from build123d import *

# Parameters (mm, degrees)
BORE_DEPTH           = 23.338105056
BORE_DEPTH_BACK      = 23.338105056
SKETCH2_R            = 6.35
RETAINING_HOLE_2_R   = 1.6891
RETAINING_HOLE_DEPTH = 23.338105056
ID_FILLET_R          = 0.254
OD_CHAMFER_SIZE      = 0.254
O_RINGS_2_W          = 1.49225
O_RINGS_2_H          = 1.666875


with BuildPart() as part:
    # Sketch1 → Bearing (revolve)
    with BuildSketch(Plane(origin=(0, 0, 0), x_dir=(0, 0, -1), z_dir=(1, 0, 0)), mode=Mode.PRIVATE) as bearing_sk:
        Polygon((-15.875, 0), (15.875, 0), (15.875, -11.1125), (12.3063, -11.1125), (12.3063, -10.00125), (11.1125, -10.00125), (11.1125, -11.1125), (-11.1125, -11.1125), (-11.1125, -10.00125), (-12.3063, -10.00125), (-12.3063, -11.1125), (-15.875, -11.1125), align=None)
    revolve(bearing_sk.sketch.rotate(Axis((0, 0, 15.875), (0, 0, -1)), 270), axis=Axis((0, 0, 15.875), (0, 0, -1)))

    # Sketch2 → Bore (cut, two sides: drawn at the far end of the back side and taken through both)
    with BuildSketch(Plane.XY.offset(-BORE_DEPTH_BACK)):
        Circle(SKETCH2_R)
    extrude(amount=BORE_DEPTH + BORE_DEPTH_BACK, mode=Mode.SUBTRACT)

    # Retaining Hole 2 → Retaining Hole (cut, through all)
    with BuildSketch(Plane(origin=(0, 0, 0), x_dir=(0, 0, -1), z_dir=(1, 0, 0))):
        with Locations(Location((0, 0, 0), (0, 0, 180))):
            Circle(RETAINING_HOLE_2_R)
    extrude(amount=RETAINING_HOLE_DEPTH, mode=Mode.SUBTRACT)

    # ID Fillet
    id_fillet_edges = [part.edges().sort_by_distance(p)[0] for p in [
        (-6.35, 0, -15.875),
        (-6.35, 0, 15.875),
    ]]
    fillet(id_fillet_edges, radius=ID_FILLET_R)

    # OD Chamfer
    od_chamfer_edges = [part.edges().sort_by_distance(p)[0] for p in [
        (-11.1125, 0, 15.875),
        (-11.1125, 0, -15.875),
    ]]
    chamfer(od_chamfer_edges, length=OD_CHAMFER_SIZE)

    # O-Rings 2 → O-Rings (revolve, cut)
    with BuildSketch(Plane(origin=(0, 0, 0), x_dir=(0, 0, -1), z_dir=(1, 0, 0)), mode=Mode.PRIVATE) as o_rings_sk:
        with Locations((-6.969125, -10.2790625)):
            Rectangle(O_RINGS_2_W, O_RINGS_2_H)
        with Locations((6.969125, -10.2790625)):
            Rectangle(O_RINGS_2_W, O_RINGS_2_H)
    revolve(o_rings_sk.sketch.rotate(Axis((0, 0, 15.875), (0, 0, -1)), 270), axis=Axis((0, 0, 15.875), (0, 0, -1)), mode=Mode.SUBTRACT)


solid = part.part
The model under review builds one solid part; all positions refer to its coordinate system, in mm. A direction names the side the tool comes from. Round coordinates to 2 decimals unless told otherwise and drop trailing zeros. Answer as a JSON object with one key per item and string values.
1. To check wall thickness, follow line 1 along Z through (x, y) = (4.25, 8.75) (3 decimals); line 2 along Z through (x, y) = (2.75, 10) (1 decimal); line 3 along Y through (x, z) = (0.25, -7). State the ranges of each line that lie inside material, in increasing order.
Results found:
{"line 1": "z = -15.875 to -7.715, -6.223 to 6.223, 7.715 to 15.875", "line 2": "z = -15.9 to -12.3, -11.1 to -7.7, -6.2 to 6.2, 7.7 to 11.1, 12.3 to 15.9", "line 3": "y = -9.44 to -6.35, 6.35 to 9.44"}
2. Machinability: for faces 4 (the face through (5.974, -9.37, 9.438)), 5 (the face through (-5, 8.2, 6.223)), 6 (the face through (8.58, 1.5, 0.78)), which of the approach directions +Z, -Z, +X, -X, +Y, -Y give a long, thin tool a straight path to every point of the face, cutting with its end or side? Answer none if there is none.
Results found:
{"face 4": "+Z, -Z", "face 5": "none", "face 6": "+X"}
3. Clearance check with flat-ended pins moving along their axes: pin 1 (8 mm diameter, centred on y = -3.5, z = -7.5, fed in from +X); pin 2 (6 mm diameter, centred on x = -3.5, z = 6, fed in from +Y); pin 3 (1.5 mm diameter, centred on x = 4, z = 8.5, fed in from +Y); pin 4 (1.5 mm diameter, centred on x = -8.5, z = 11, fed in from +Y). State where each tip first meets the part, or that it passes through.
Results found:
{"pin 1": "stops at x = 11.11", "pin 2": "stops at y = 11.1", "pin 3": "stops at y = 10.63", "pin 4": "stops at y = 7.96"}
4. The part is to be moulded in two halves that separate along Z. For faces 1 (the face through (-5, 5, -15.875)), 2 (the face through (5.974, -9.37, -13.94)), 3 (the face through (-5, 8.2, 7.715)), say which applies: pulls with the +Z half, pulls with the -Z half, needs draft (parallel to the pull), parting line crosses it, or undercut.
Results found:
{"face 1": "pulls with the -Z half", "face 2": "needs draft", "face 3": "undercut"}
5. We need section A-A on y = 0. State how many separate pieces and enclosed holes the cut face has, and give its area (3 significant figures).
Results found:
{"separate pieces": "3", "enclosed holes": "0", "area": "271 mm^2"}
